Read the model definition and answer for the solid it produces. Units are mm, in the model's axes. A direction names the side the tool comes from. Coordinates: 2 decimals unless noted, no trailing zeros. Loops run counter-clockwise (first coordinate to the right, second up) from the corner with the lowest first, then second, coordinate; pieces in that order, holes last.
Q1. Section A-A (z = -30) is taken. Give the vertices of the cut face in (x, y), then the cut area to 3 significant figures.
Q2. Straight lines are drawn through the part: line 1 (Z direction, x = 0, y = 4.5); line 2 (Z direction, x = 12, y = 44); line 3 (Y direction, x = 0, z = 21). For each, find the intervals that lie inside material, in ascending order.
Q3. Section D-D (z = 0) is taken. Give the vertices of the cut face in (x, y).
Q4. Flat-ended cylindrical pins translate along their axes: P1, Ø2, axis at y = 33.5, z = 24.5, coming from the -X side; P2, Ø22, axis at y = 46, z = 23.5, coming from the +X side; P3, Ø4, axis at x = -1, z = 21.5, coming from the +Y side. Find the tip coordinate at first contact, or state that the pin passes through.
Q5. The mould has two halves that part along X. Classify faces 4 (the face through (7, 45, 15)), 5 (the face through (0, 10, 0)), 6 (the face through (-5.42, 45.594, -24.86)), 7 (the face through (30, 47, 25)): pulls with the +X half, pulls with the -X half, needs draft (parallel to the pull), parting line crosses it, or undercut.
Q6. Which of the six approach directions +Z, -Z, +X, -X, +Y, -Y give full straight-line access (tool end or side, diameter ignored) to faces 1 (the face through (-7, 45, 35)), 2 (the face through (23.846, 4.93, 7.509)), 3 (the face through (-30, 47, -25))?
Q7. Section C-C (y = 83.5) is taken. Give the vertices of the cut face in (x, z).
Q8. Section B-B (x = 10) is taken. Give the vertices of the cut face in (y, z).
Autodesk Inventor part; units mm, degrees
ref_plane "YZ Plane" through (0, 0, 0) normal (1, 0, 0) x (0, 1, 0)
ref_plane "XZ Plane" through (0, 0, 0) normal (0, 1, 0) x (-1, 0, 0)
ref_plane "XY Plane" through (0, 0, 0) normal (0, 0, 1) x (1, 0, 0)
sketch "Sketch1" plane through (0, 0, 0) normal (0, 1, 0) x (-1, 0, 0)
  circle A0 centre (0, 0) radius 50
  dimension "d0" = 100
extrude "Extrusion1" add sketch "Sketch1" along normal blind 25
sketch "Sketch2" plane through (0, 0, 0) normal (0, -1, 0) x (1, 0, 0)
  circle A0 centre (0, 0) radius 25
  dimension "d3" = 50
extrude "Extrusion2" cut sketch "Sketch2" against normal blind 10
sketch "Sketch3" plane through (0, 25, 0) normal (0, 1, 0) x (1, 0, 0)
  line L0 (-30, -35) -> (30, -35)
  line L1 (30, -35) -> (30, 35)
  line L2 (30, 35) -> (-30, 35)
  line L3 (-30, 35) -> (-30, -35)
  line L4 (-30, -35) -> (30, 35) construction
  line L5 (30, -35) -> (-30, 35) construction
  line L6 (-30, -35) -> (30, -35)
  line L7 (30, -35) -> (30, -15)
  line L8 (30, -15) -> (-30, -15)
  line L9 (-30, -15) -> (-30, -35)
  line L10 (-30, 35) -> (30, 35)
  line L11 (30, 35) -> (30, 15)
  line L12 (30, 15) -> (-30, 15)
  line L13 (-30, 15) -> (-30, 35)
  point P0 (0, 0)
  dimension "d6" = 60
  dimension "d7" = 70
  dimension "d8" = 20
  dimension "d9" = 20
extrude "Extrusion3" add sketch "Sketch3" along normal blind 75 contours L3 L8 L1 L0 | L3 L2 L1 L12
sketch "Sketch4" plane through (-30, 25, 35) normal (0, 0, 1) x (1, 0, 0)
  line L0 (60, 0) -> (60, 75)
  circle A0 centre (30, 45) radius 30
  line L1 (0, 75) -> (60, 75)
  line L2 (60, 0) -> (60, 75)
  circle A1 centre (30, 45) radius 25
  line L3 (0, 45) -> (0, 75)
  line L4 (60, 75) -> (60, 45)
  point P0 (30, -25)
  point P1 (30, 75)
  dimension "d12" = 60
  dimension "d13" = 50
extrude "Extrusion4" cut sketch "Sketch4" against normal blind 100 contours A0 L1 L0 | L3 L1 A0 | A1
properties part number "JOINT BASE2"
Numbers:
1. outline: (-40, 0) - (40, 0) - (40, 25) - (30, 25) - (30, 70) arc R30 ccw to (-30, 70) - (-30, 25) - (-40, 25) - close; hole circle Ø50 at (0, 70)
1. area: 4,150 mm2
2. line 1: z = -50 to -25, 25 to 50
2. line 2: z = -35 to -15, 15 to 35
2. line 3: y = 10 to 45, 95 to 100
3. outline: (-50, 0) - (-25, 0) - (-25, 10) - (25, 10) - (25, 0) - (50, 0) - (50, 25) - (-50, 25) - close
4. P1: stops at x = -30
4. P2: stops at x = 30
4. P3: stops at y = 100
5. face 4: needs draft
5. face 5: undercut
5. face 6: undercut
5. face 7: pulls with the +X half
6. face 1: +Z, +X, -X, +Y
6. face 2: -Y
6. face 3: +Z, -Z, -X, +Y
7. outline: (-26.79, -35) - (-21.04, -35) - (-21.04, -15) - (-26.79, -15) - close; (-26.79, 15) - (-21.04, 15) - (-21.04, 35) - (-26.79, 35) - close; (21.04, -35) - (26.79, -35) - (26.79, -15) - (21.04, -15) - close; (21.04, 15) - (26.79, 15) - (26.79, 35) - (21.04, 35) - close
8. outline: (0, -48.99) - (25, -48.99) - (25, -35) - (47.09, -35) - (47.09, -15) - (25, -15) - (25, 15) - (47.09, 15) - (47.09, 35) - (25, 35) - (25, 48.99) - (0, 48.99) - (0, 22.91) - (10, 22.91) - (10, -22.91) - (0, -22.91) - close; (92.91, -35) - (98.28, -35) - (98.28, -15) - (92.91, -15) - close; (92.91, 15) - (98.28, 15) - (98.28, 35) - (92.91, 35) - close
